Work out the finished part from the listing and answer in its coordinate system (mm). Face numbers are marked on the shaded views. A direction names the side the tool comes from. Give positions to 0.01 mm unless a question says otherwise; leave off trailing zeros. Order: outer loops, then holes, each group sorted by start corner. A loop starts at its lowest first (then second) coordinate and runs counter-clockwise, first axis right, second up. Notation, with made-up numbers: M 0.5,44.5 L 4.5,44.5 A25 cw 4.5,71.5 Z; hole C -4.75,16 d8. An arc over 180 degrees is marked long. One line per item, written item: value.
from build123d import *

# Parameters (mm, degrees)
BOSS_EXTRUDE1_DEPTH  = 12
SKETCH2_R            = 9
BOSS_EXTRUDE2_DEPTH  = 6
BOSS_EXTRUDE7_DEPTH  = 8
BOSS_EXTRUDE8_START  = -8
BOSS_EXTRUDE8_DEPTH  = 8
BOSS_EXTRUDE9_START  = -8
BOSS_EXTRUDE9_DEPTH  = 4
BOSS_EXTRUDE11_DEPTH = 21.5
BOSS_EXTRUDE12_DEPTH = 25
CHAMFER1_SIZE        = 10
SKETCH8_R            = 1.7000000000000015
CUT_EXTRUDE1_DEPTH   = 84.10385069297331
CHAMFER2_SIZE        = 3
FILLET1_R            = 2
FILLET2_3_ANGLE      = 270
BOSS_EXTRUDE13_DEPTH = 20
CUT_EXTRUDE2_DEPTH   = 101.54294892174786
SKETCH11_R           = 1.7000000000000037
CUT_EXTRUDE3_DEPTH   = 105.74850838221995
CHAMFER3_SIZE        = 1
CUT_EXTRUDE5_DEPTH   = 15
CHAMFER4_SIZE        = 1
FILLET3_R            = 1


with BuildPart() as part:
    # Sketch1 → Boss-Extrude1 (new body)
    with BuildSketch(Plane(origin=(0, 0, 0), x_dir=(0, 0, -1), z_dir=(1, 0, 0))):
        with BuildLine():
            Line((-15, 0), (-15, 50))
            Line((-15, 50), (15, 50))
            Line((15, 50), (15, 0))
            ThreePointArc((15, 0), (-2.76e-15, -15), (-15, 0))
        make_face()
    extrude(amount=BOSS_EXTRUDE1_DEPTH)

    # Sketch2 → Boss-Extrude2 (add)
    with BuildSketch(Plane(origin=(12, 0, 0), x_dir=(0, 0, -1), z_dir=(1, 0, 0))):
        Circle(SKETCH2_R)
    extrude(amount=BOSS_EXTRUDE2_DEPTH)

    # Sketch3 → Boss-Extrude7 (add)
    with BuildSketch(Plane(origin=(18.000000000000004, 0, 0), x_dir=(0, 0, -1), z_dir=(1, 0, 0))):
        with BuildLine():
            Line((-4, 0), (0, 0))
            Line((0, 0), (0, 4))
            ThreePointArc((8.285e-14, 4), (-2.828427124746161, 2.828427124746219), (-4, 4.9e-16))
        make_face()
        with BuildLine():
            Line((0, 4), (0, 0))
            Line((0, 0), (-4, 0))
            ThreePointArc((-4, 4.9e-16), (-7.3e-16, -4), (4, -9.8e-16))
            ThreePointArc((4, 0), (2.8284271247462196, 2.828427124746161), (8.285e-14, 4))
        make_face()
    extrude(amount=BOSS_EXTRUDE7_DEPTH)

    # Sketch5 → Boss-Extrude8 (add)
    with BuildSketch(Plane(origin=(26.000000000000004, 0, 0), x_dir=(0, 0, -1), z_dir=(1, 0, 0)).offset(BOSS_EXTRUDE8_START)):
        with BuildLine():
            Line((-9, 0), (-6.000000000000001, 0))
            ThreePointArc((-6.000000000000001, 7.3e-16), (-5.605034153776295, 2.140932538638541), (-4.4721359549995805, 3.9999999999999996))
            Line((-4.472135954999581, 4), (-8.06225774829855, 4))
            ThreePointArc((-8.062257748298551, 4), (-8.762428879445668, 2.054224946946299), (-9, 1.1e-16))
        make_face()
        with BuildLine():
            Line((-6.708203932499368, 6), (0, 6))
            Line((0, 6), (0, 9))
            ThreePointArc((0, 9), (-3.6742346141747673, 8.215838362577493), (-6.7082039324993685, 6.000000000000003))
        make_face()
    extrude(amount=BOSS_EXTRUDE8_DEPTH)

    # Sketch5_3 → Boss-Extrude9 (add)
    with BuildSketch(Plane(origin=(26.000000000000004, 0, 0), x_dir=(0, 0, -1), z_dir=(1, 0, 0)).offset(BOSS_EXTRUDE9_START)):
        with BuildLine():
            Line((-8.06225774829855, 4), (-4.472135954999581, 4))
            ThreePointArc((-4.4721359549995805, 3.9999999999999996), (-2.4494897427831788, 5.477225575051661), (3.7e-16, 6.000000000000001))
            Line((0, 6), (-6.708203932499368, 6))
            ThreePointArc((-6.7082039324993685, 6.000000000000003), (-7.452626018121394, 5.045628348780764), (-8.062257748298551, 4))
        make_face()
    extrude(amount=BOSS_EXTRUDE9_DEPTH)

    # Sketch6 → Boss-Extrude11 (add)
    with BuildSketch(Plane.ZY):
        Polygon((-15, 50), (15, 50), (15, 42), (-14.999999999999998, 42), align=None)
    extrude(amount=BOSS_EXTRUDE11_DEPTH)

    # Sketch7 → Boss-Extrude12 (add)
    with BuildSketch(Plane(origin=(0, 50, 0), x_dir=(1, 0, 0), z_dir=(0, 1, 0))):
        Polygon((-21.5, 15), (-6.499999999999999, 15), (-6.499999999999996, -15), (-21.5, -15), align=None)
    extrude(amount=BOSS_EXTRUDE12_DEPTH)

    # Chamfer1
    chamfer1_edges = [part.edges().sort_by_distance(p)[0] for p in [
        (-6.499999999999997, 50, 0),
    ]]
    chamfer(chamfer1_edges, length=CHAMFER1_SIZE)

    # Sketch8 → Cut-Extrude1 (cut, through all)
    with BuildSketch(Plane(origin=(-6.499999999999997, 0, 7.5e-16), x_dir=(-1.2e-16, 0, -1), z_dir=(1, 0, -1.2e-16))):
        with Locations((-9.999999999999998, 66.00000000000007)):
            Circle(SKETCH8_R)
        with Locations(Location((9.999999999999998, 66.00000000000007, 0), (0, 0, 180))):
            Circle(SKETCH8_R)
    extrude(amount=-CUT_EXTRUDE1_DEPTH, mode=Mode.SUBTRACT)

    # Chamfer2
    chamfer2_edges = [part.edges().sort_by_distance(p)[0] for p in [
        (12, 50, 0),
        (12, 25, 15),
        (12, -14.999999999999998, -2.03e-15),
        (0, 21, -15),
        (0, 21, 15),
        (0, -14.999999999999998, -2.03e-15),
        (0, 42, 0),
        (-10.75, 42, -14.999999999999998),
        (-10.75, 42, 15),
        (12, 25, -15),
    ]]
    chamfer(chamfer2_edges, length=CHAMFER2_SIZE)

    # Fillet1
    fillet1_edges = [part.edges().sort_by_distance(p)[0] for p in [
        (-13.999999999999996, 75, 15),
        (-6.499999999999997, 75, 0),
        (-14, 75, -15),
    ]]
    fillet(fillet1_edges, radius=FILLET1_R)

    # Fillet2: read off the stored shape, not the designer's step
    # Fillet2 outline → Fillet2 (revolve, cut)
    with BuildSketch(Plane.YX):
        with BuildLine():
            ThreePointArc((3, 26), (3.707106781, 25.707106781), (4, 25))
            Line((4, 25), (4, 26))
            Line((4, 26), (3, 26))
        make_face()
    revolve(axis=Axis((0, 0, 0), (1, 0, 0)), mode=Mode.SUBTRACT)

    # Fillet2 2 outline → Fillet2 2 (revolve)
    with BuildSketch(Plane.YX):
        with BuildLine():
            ThreePointArc((10, 12), (9.292893219, 12.292893219), (9, 13))
            Line((9, 13), (9, 12))
            Line((9, 12), (10, 12))
        make_face()
    revolve(axis=Axis((0, 0, 0), (1, 0, 0)))

    # Fillet2 3 outline → Fillet2 3 (revolve, cut)
    with BuildSketch(Plane.ZX):
        with BuildLine():
            ThreePointArc((8, 18), (8.707106781, 17.707106781), (9, 17))
            Line((9, 17), (9, 18))
            Line((9, 18), (8, 18))
        make_face()
    revolve(axis=Axis((0, 0, 0), (1, 0, 0)), revolution_arc=FILLET2_3_ANGLE, mode=Mode.SUBTRACT)

    # Sketch9 → Boss-Extrude13 (add)
    with BuildSketch(Plane(origin=(0, 75.00000000000001, 0), x_dir=(1, 0, 0), z_dir=(0, 1, 0))):
        Polygon((-15.500000000000007, -1.041e-14), (-18.500000000000004, 5.1961524227066205), (-21.5, 5.1961524227066205), (-21.5, -5.196152422706621), (-18.5, -5.196152422706619), align=None)
    extrude(amount=BOSS_EXTRUDE13_DEPTH)

    # Sketch10 → Cut-Extrude2 (cut, through all)
    with BuildSketch(Plane.XY.offset(5.196152422706602)):
        with BuildLine():
            Line((-21.5, 86.70000000000002), (-21.5, 83.30000000000003))
            ThreePointArc((-21.5, 83.30000000000003), (-19.80000000000001, 85.00000000000001), (-21.5, 86.70000000000002))
        make_face()
    extrude(amount=-CUT_EXTRUDE2_DEPTH, mode=Mode.SUBTRACT)

    # Sketch11 → Cut-Extrude3 (cut, through all)
    with BuildSketch(Plane(origin=(-15.500000000000007, 0, 1.79e-15), x_dir=(-1.2e-16, 0, -1), z_dir=(1, 0, -1.2e-16))):
        with Locations(Location((-8.62e-15, 85.00000000000001, 0), (0, 0, 90))):
            Circle(SKETCH11_R)
    extrude(amount=-CUT_EXTRUDE3_DEPTH, mode=Mode.SUBTRACT)

    # Chamfer3
    chamfer3_edges = [part.edges().sort_by_distance(p)[0] for p in [
        (-17.000000000000004, 75.00000000000001, 2.5980762113533147),
        (-17.000000000000007, 75.00000000000001, -2.5980762113533054),
        (-20, 75.00000000000001, -5.1961524227066205),
        (-20, 75.00000000000001, 5.19615242270662),
    ]]
    chamfer(chamfer3_edges, length=CHAMFER3_SIZE)

    # Sketch12 → Cut-Extrude5 (cut)
    with BuildSketch(Plane.ZY):
        Polygon((6.200000000000001, 8.7e-16), (3.100000000000001, 5.369357503463521), (-3.100000000000001, 5.369357503463522), (-6.200000000000002, 1.74e-15), (-3.100000000000001, -5.3693575034635215), (3.0999999999999996, -5.369357503463523), align=None)
    extrude(amount=-CUT_EXTRUDE5_DEPTH, mode=Mode.SUBTRACT)

    # Chamfer4
    chamfer4_edges = [part.edges().sort_by_distance(p)[0] for p in [
        (0, -2.684678751731761, 4.65),
        (0, 2.6846787517317607, 4.650000000000001),
        (0, 5.3693575034635215, 0),
        (0, 2.684678751731762, -4.650000000000002),
        (0, -2.68467875173176, -4.650000000000001),
        (0, -5.369357503463522, -4.4e-16),
    ]]
    chamfer(chamfer4_edges, length=CHAMFER4_SIZE)

    # Fillet3
    fillet3_edges = [part.edges().sort_by_distance(p)[0] for p in [
        (26.000000000000004, 0, 7.5),
        (26.000000000000004, 2.054224946946299, 8.762428879445668),
        (26.000000000000004, 7.5, 0),
        (26.000000000000004, 8.215838362577493, 3.674234614174768),
    ]]
    fillet(fillet3_edges, radius=FILLET3_R)


solid = part.part
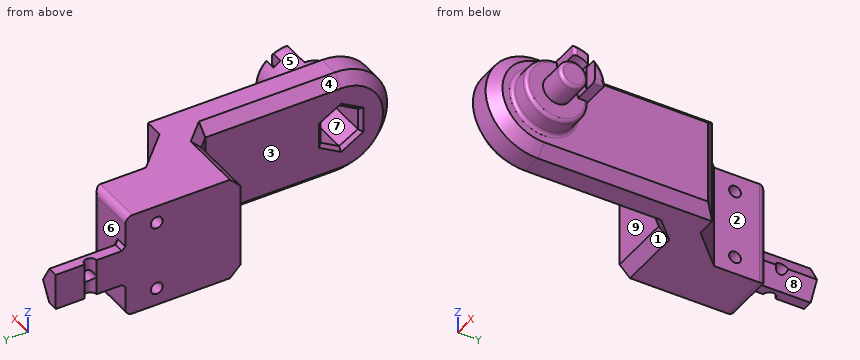
(1) Which of the six approach directions +Z, -Z, +X, -X, +Y, -Y give full straight-line access (tool end or side, diameter ignored) to the marked faces 1, 2, 3, 4 and 5?
Findings:
face 1: -Z, -X, -Y
face 2: +Z, -Z, +X, +Y
face 3: +Z, -Z, -X, -Y
face 4: +Z, -X, -Y
face 5: +X
(2) Given P1, Ø8, axis at y = 35.5, z = -6.5, coming from the +X side; P2, Ø6, axis at x = 5.5, z = 2, coming from the +Y side; P3, Ø5, axis at x = 9.5, z = 1.5, coming from the +Y side; P4, Ø3, axis at y = 66, z = -10, coming from the -X side, each flat-ended and moving along its own axis, determine where each tip first touches the part or whether it passes through.
Findings:
P1: stops at x = 12
P2: stops at y = 51
P3: stops at y = 50
P4: passes through
(3) Section D-D, the plane y = 85 is taken. Give the vertices of the cut face in (x, z).
Findings:
outline: M -19.8,-5.2 L -18.5,-5.2 L -16.48,-1.7 L -19.8,-1.7 Z; M -19.8,1.7 L -16.48,1.7 L -18.5,5.2 L -19.8,5.2 Z
(4) Section C-C, the plane x = -11 is taken. Give the vertices of the cut face in (y, z), then the cut area to 3 significant figures.
Findings:
outline: M 42,-12 L 45,-15 L 73,-15 A2 ccw 75,-13 L 75,13 A2 ccw 73,15 L 45,15 L 42,12 Z; hole C 66,-10 d3.4; hole C 66,10 d3.4
area: 961 mm^2
(5) Section B-B, the plane x = 6.5 is taken. Give the vertices of the cut face in (y, z).
Findings:
outline: M 0,-15 L 50,-15 L 50,15 L 0,15 A15 ccw Z; hole M -5.37,-3.1 L 0,-6.2 L 5.37,-3.1 L 5.37,3.1 L 0,6.2 L -5.37,3.1 Z
(6) Find the intervals of material crossed by probe 1 along Y at (x, z) = (-15.5, -10); probe 2 along Z at (x, y) = (-19.25, 85); probe 3 along X at (y, z) = (-1.5, -2), in increasing order. Write a range as from..to.
Findings:
probe 1: y = 42..64.3, 67.7..75
probe 2: z = -5.2..-1.7, 1.7..5.2
probe 3: x = 15..26
(7) Determine the mould class of the marked faces 6, 7, 8 and 9 for opening direction Y: pulls with the +Y half, pulls with the -Y half, needs draft (parallel to the pull), parting line crosses it, or undercut.
Findings:
face 6: pulls with the +Y half
face 7: undercut
face 8: needs draft
face 9: pulls with the -Y half
(8) Section A-A, the plane y = 66 is taken. Give the vertices of the cut face in (x, z), then the cut area to 3 significant figures.
Findings:
outline: M -21.5,-15 L -6.5,-15 L -6.5,-11.7 L -21.5,-11.7 Z; M -21.5,-8.3 L -6.5,-8.3 L -6.5,8.3 L -21.5,8.3 Z; M -21.5,11.7 L -6.5,11.7 L -6.5,15 L -21.5,15 Z
area: 348 mm^2
